Design review of the part built by this model. Coordinates are the model's own, in mm. A direction names the side the tool comes from. Coordinates: 2 decimals unless noted, no trailing zeros. Order: outer loops, then holes, each group sorted by start corner. A loop starts at its lowest first (then second) coordinate and runs counter-clockwise, first axis right, second up. Notation, with made-up numbers: (-26, 13.25) - (-6, 13.25) arc R22 ccw to (-6, 31.25) - close; hole circle Ø10 at (-26, -39.75). An arc over 180 degrees is marked (long way). Write each question's results on one line, items separated by ' | '. Start each with the question number.
```python
from build123d import *

# Parameters (mm, degrees)
F0_W     = 89.496315
F0_H     = 98.643005
F1_DEPTH = 20
F2_W     = 22.195481
F2_H     = 63.440859
F3_DEPTH = 25


with BuildPart() as f1:
    # F0 (on Top) → F1 (new body)
    with BuildSketch(Plane.XY):
        with Locations((3.052593, -2.165347)):
            Rectangle(F0_W, F0_H)
    extrude(amount=F1_DEPTH)

    # F2 (on Front) → F3 (join)
    with BuildSketch(Plane.XZ):
        with Locations((-29.008787, 31.720429)):
            Rectangle(F2_W, F2_H)
    extrude(amount=F3_DEPTH)


solid = f1.part
```
(1) Take a section at C-C (z = 32). State the section outline as (x, y) points, plus the area to 3 significant figures.
(2) Take a section at D-D (y = -38.5). State the section outline as (x, z) points.
(3) Take a section at A-A (y = -21.5). State the section outline as (x, z) points, plus the area to 3 significant figures.
(4) Clearance check with flat-ended pins moving along their axes: pin 1 (6 mm diameter, centred on y = -17.5, z = 21, fed in from +X); pin 2 (5 mm diameter, centred on y = -12.5, z = 31.5, fed in from -X); pin 3 (8 mm diameter, centred on y = -8.5, z = 36, fed in from +X); pin 4 (3 mm diameter, centred on x = -21.5, z = 37, fed in from -Y). State where each tip first meets the part, or that it passes through.
(5) To check wall thickness, follow line 1 along Z through (x, y) = (37.5, -29.5); line 2 along X through (y, z) = (-1.5, 51.5); line 3 along Y through (x, z) = (-35, 43.5). State the ranges of each line that lie inside material, in increasing order. Write a range as [from, to].
(6) Tool access review of faces 1 (the face through (-17.911, -12, 41)), 2 (the face through (-40.107, -12, 41)), 3 (the face through (-29, 0, 42)): name each direction out of +Z, -Z, +X, -X, +Y, -Y from which nothing blocks a thin tool from reaching the whole face with its end or side.
(7) Take a section at B-B (x = -20.5). State the section outline as (y, z) points.
Worked out:
1) outline: (-40.11, -25) - (-17.91, -25) - (-17.91, 0) - (-40.11, 0) - close | area: 555 mm^2
2) outline: (-41.7, 0) - (47.8, 0) - (47.8, 20) - (-41.7, 20) - close
3) outline: (-41.7, 0) - (47.8, 0) - (47.8, 20) - (-17.91, 20) - (-17.91, 63.44) - (-40.11, 63.44) - (-40.11, 20) - (-41.7, 20) - close | area: 2,750 mm^2
4) pin 1: x = 47.8 | pin 2: x = -40.11 | pin 3: x = -17.91 | pin 4: y = -25
5) line 1: [0, 20] | line 2: [-40.11, -17.91] | line 3: [-25, 0]
6) face 1: +Z, +X, +Y, -Y | face 2: +Z, -X, +Y, -Y | face 3: +Z, +X, -X, +Y
7) outline: (-51.49, 0) - (47.16, 0) - (47.16, 20) - (0, 20) - (0, 63.44) - (-25, 63.44) - (-25, 20) - (-51.49, 20) - close
